Model file for the job. Use its own axes, mm. A direction names the side the tool comes from. Round coordinates to 2 decimals unless told otherwise and drop trailing zeros. Order: outer loops, then holes, each group sorted by start corner. A loop starts at its lowest first (then second) coordinate and runs counter-clockwise, first axis right, second up. Notation, with made-up numbers: (-38, 56.5) -> (8, 56.5) arc R24 cw to (8, 94.5) -> close; hole circle Ø5 at (34, 0). An arc over 180 degrees is marked (long way). Put each result on its own line as item: value. Start each with the question number.
Q1. Probe L1, parallel to Y at x = -0.75, z = 15; L2, parallel to Y at x = -1.1, z = 15; L3, parallel to Z at x = 2.5, y = -12. List the from-to ranges inside material, lowest first.
Q2. Cut at D-D, the plane y = 11.5. List the corners of the cut face in (x, z).
Q3. Cut at B-B, the plane z = 4.5. List the corners of the cut face in (x, y), and give its area (3 significant figures).
Q4. Flat gauge pins, fed straight in: P1, Ø6, axis at x = 12.5, z = 18, coming from the +Y side; P2, Ø4, axis at x = 14, z = 10.5, coming from the +Y side; P3, Ø4, axis at x = 7, z = 16.5, coming from the +Y side. Where does each tip first touch, or does it go through?
Q5. Pull direction Z, two halves, no side cores. Call faces 4 (the face through (5, -6, 0)), 5 (the face through (0, -40, 15)), 6 (the face through (5, -6, 30)), 7 (the face through (0.028, -31.108, 17.064)): released by +Z, released by -Z, zero draft, split by the parting line, or undercut.
Q6. 3-axis set-ups, long thin cutter, end or side, ignore diameter. For faces 1 (the face through (5.84, 4.09, 15.1)), 2 (the face through (2, 27, 15)), 3 (the face through (2, -37, 15)): which of +Z, -Z, +X, -X, +Y, -Y reach the whole face in a straight line?
Q7. Cut at C-C, the plane z = 15. List the corners of the cut face in (x, y).
Q8. Cut at A-A, the plane y = 33. List the corners of the cut face in (x, z), and give its area (3 significant figures).
Autodesk Inventor part; units mm, degrees
ref_plane "Work Plane6" through (-19.9203, -6.9203, 0) normal (0.7071, 0.7071, 0) x (-0.7071, 0.7071, 0)
ref_plane "YZ Plane" through (0, 0, 0) normal (1, 0, 0) x (0, 1, 0)
ref_plane "XZ Plane" through (0, 0, 0) normal (0, 1, 0) x (-1, 0, 0)
sketch "Sketch6" plane through (0, 0, 0) normal (0, 0, 1) x (1, 0, 0)
  line L0 (-2, -40) -> (2, -40)
  line L1 (2, -40) -> (2, 40)
  line L2 (2, 40) -> (-2, 40)
  line L3 (-2, 40) -> (-2, -40)
  line L4 (-2, -40) -> (2, 40) construction
  line L5 (2, -40) -> (-2, 40) construction
  line L6 (2, 15) -> (23.2132, -6.2132)
  line L7 (2, 15) -> (32, 15) construction
  line L8 (23.2132, -6.2132) -> (2, -27.4264)
  line L9 (2, -27.4264) -> (2, 15)
  point P0 (0, 0)
  point P1 (2, -27.4264)
  dimension "d23" = 4
  dimension "d24" = 80
  dimension "d25" = 30
  dimension "d26" = 45
  dimension "d27" = 30
  dimension "d28" = 90
  dimension "d29" = 25
extrude "Extrusion6" add sketch "Sketch6" along normal blind 30
sketch "Sketch7" plane through (2, 15, 0) normal (0.7071, 0.7071, 0) x (-0.7071, 0.7071, 0)
  circle A0 centre (-15, 15) radius 4.4
  line L0 (-30, 0) -> (-30, 30)
  line L1 (-30, 30) -> (0, 30)
  point P0 (-9.1924, 0)
  dimension "d32" = 15
  dimension "d33" = 15
  dimension "d34" = 8.8
extrude "Extrusion7" cut sketch "Sketch7" against normal blind 27.5
ref_plane "Work Plane6" through (-19.9203, -6.9203, 0) normal (0.7071, 0.7071, 0) x (-0.7071, 0.7071, 0)
sketch "Sketch8" plane through (-19.9203, -6.9203, 0) normal (0.7071, 0.7071, 0) x (-0.7071, 0.7071, 0)
  circle A0 centre (-15, 15) radius 4.4
  circle A1 centre (-15, 15) radius 7
  point P0 (-9.1924, 0)
  dimension "d38" = 14
extrude "Extrusion8" cut sketch "Sketch8" along normal blind 26 contours A0 | A1
sketch "Sketch9" plane through (2, -40, 0) normal (1, 0, 0) x (0, 0, -1)
  circle A0 centre (-15, 7) radius 2.8
  line L0 (0, 0) -> (-30, 0)
  line L1 (-30, 0) -> (-30, 12.5736)
  circle A1 centre (-15, 73) radius 2.8
  line L2 (0, 55) -> (0, 80)
  line L3 (0, 80) -> (-30, 80)
  point P0 (0, 40)
  dimension "d41" = 5.6
  dimension "d42" = 7
  dimension "d43" = 15
  dimension "d46" = 15
  dimension "d47" = 7
extrude "Extrusion9" cut sketch "Sketch9" against normal through all
properties part number "45bracket" material "Acetal Resin, Black"
Ans:
1. L1: y = -40 to -35.8, -30.2 to -18.86, 0.94 to 30.2, 35.8 to 40
1. L2: y = -40 to -35.8, -30.2 to -19.21, 0.59 to 30.2, 35.8 to 40
1. L3: z = 0 to 9.59, 20.41 to 30
2. outline: (-2, 0) -> (5.5, 0) -> (5.5, 30) -> (-2, 30) -> close
3. outline: (-2, -40) -> (2, -40) -> (2, -27.43) -> (23.21, -6.21) -> (2, 15) -> (2, 40) -> (-2, 40) -> close
3. area: 770 mm^2
4. P1: stops at y = 7.5
4. P2: stops at y = 5
4. P3: stops at y = 12
5. face 4: released by -Z
5. face 5: zero draft
5. face 6: released by +Z
5. face 7: undercut
6. face 1: none
6. face 2: +Z, -Z, +X, +Y
6. face 3: +Z, -Z, +X, -Y
7. outline: (-2, -40) -> (2, -40) -> (2, -35.8) -> (-2, -35.8) -> close; (-2, -30.2) -> (2, -30.2) -> (2, -27.43) -> (23.21, -6.21) -> (15.72, 1.28) -> (12.18, -2.25) -> (14.02, -4.09) -> (-2, -20.11) -> close; (-2, -0.31) -> (4.12, 5.81) -> (5.96, 3.97) -> (9.5, 7.5) -> (2, 15) -> (2, 30.2) -> (-2, 30.2) -> close; (-2, 35.8) -> (2, 35.8) -> (2, 40) -> (-2, 40) -> close
8. outline: (-2, 0) -> (2, 0) -> (2, 12.2) -> (-2, 12.2) -> close; (-2, 17.8) -> (2, 17.8) -> (2, 30) -> (-2, 30) -> close
8. area: 97.6 mm^2
